Part model, mm, in its own coordinate system. Round coordinates to 2 decimals unless told otherwise and drop trailing zeros. Write each loop counter-clockwise with the first axis right and the second up, starting at its lowest first coordinate (ties: lowest second). Pieces come first, ordered by that corner, then holes. Notation, with made-up numbers: M 32,83 L 58,83 A27 ccw 58,119 Z; hole C -39,-8.5 d6. An arc over 180 degrees is marked long. One line per question, with ' | ' between items. Start each with the question number.
1) Saw through at B-B (y = 0). List the corners of the cut face in (x, z), plus the area to 3 significant figures.
2) Drop flat-ended pins along their axis: pin 1 Ø3 at (x, y) = (0.5, 2) entering from +Z; pin 2 Ø2 at (y, z) = (-1.5, -16.5) entering from +X; pin 3 Ø2 at (y, z) = (2, -14.5) entering from +X. Give the stop position or say it passes through.
3) Mould opens along Y. For faces 1 (the face through (-3, 0, -2)), 2 (the face through (-0.042, 0.481, -1.526)), 3 (the face through (0, -2, -15)) say: pulls with the +Y half, pulls with the -Y half, needs draft (parallel to the pull), parting line crosses it, or undercut.
4) Saw through at A-A (z = 0). List the corners of the cut face in (x, y).
5) Saw through at C-C (x = 2.5). List the corners of the cut face in (y, z).
6) Wall check: probe 1 along Y at (x, z) = (-0.95, 0); probe 2 along X at (y, z) = (0, -14); probe 3 along Y at (x, z) = (1.75, -0.5). Give the ranges that are in metal, low to high. Write a range as [from, to].
7) Saw through at D-D (x = 0). List the corners of the cut face in (y, z).
```python
from build123d import *

# Parameters (mm, degrees)
F_0012_CYLINDER_SKETCH_R     = 2
F_0012_CYLINDER_DEPTH        = 24
F_0014_CYLINDER_SKETCH_R     = 4
F_0014_CYLINDER_DEPTH        = 6
F_0014_CYLINDER_ROTATE_ANGLE = 90
F_0016_CYLINDER_SKETCH_R     = 1.6
F_0016_CYLINDER_DEPTH        = 8
F_0016_CYLINDER_ROTATE_ANGLE = 90


with BuildPart() as part:
    # 0012_cylinder_Sketch → 0012_cylinder (new body)
    with BuildSketch(Plane.XY):
        Circle(F_0012_CYLINDER_SKETCH_R)
    extrude(amount=F_0012_CYLINDER_DEPTH)


with BuildPart() as part_1:
    # 0012_cylinder_Translate: moved
    add(part.part.moved(Location((0, 0, -27))))


with BuildPart() as body_2:
    # 0014_cylinder_Sketch → 0014_cylinder (new body)
    with BuildSketch(Plane.XY):
        Circle(F_0014_CYLINDER_SKETCH_R)
    extrude(amount=F_0014_CYLINDER_DEPTH)


with BuildPart() as body_2_1:
    # 0014_cylinder_Rotate: moved
    add(body_2.part.rotate(Axis((0, 0, 0), (0, 1, 0)), F_0014_CYLINDER_ROTATE_ANGLE))


with BuildPart() as body_2_2:
    # 0014_cylinder_Translate: moved
    add(body_2_1.part.moved(Location((-3, 0, 0))))


with BuildPart() as part_2:
    add(part_1.part)

    # 0015_add: union body 2
    add(body_2_2.part)


with BuildPart() as body_2_2_1:
    # 0016_cylinder_Sketch → 0016_cylinder (new body)
    with BuildSketch(Plane.XY):
        Circle(F_0016_CYLINDER_SKETCH_R)
    extrude(amount=F_0016_CYLINDER_DEPTH)


with BuildPart() as body_2_2_2:
    # 0016_cylinder_Rotate: moved
    add(body_2_2_1.part.rotate(Axis((0, 0, 0), (0, 1, 0)), F_0016_CYLINDER_ROTATE_ANGLE))


with BuildPart() as body_2_2_3:
    # 0016_cylinder_Translate: moved
    add(body_2_2_2.part.moved(Location((-4, 0, 0))))


with BuildPart() as part_3:
    add(part_2.part)

    # 0017_sub: cut body 2 2
    add(body_2_2_3.part, mode=Mode.SUBTRACT)


solid = part_3.part
```
Answer key:
1) outline: M -3,-4 L -2,-4 L -2,-27 L 2,-27 L 2,-4 L 3,-4 L 3,-1.6 L -3,-1.6 Z; M -3,1.6 L 3,1.6 L 3,4 L -3,4 Z | area: 121 mm2
2) pin 1: stops at z = 3.97 | pin 2: stops at x = 1.94 | pin 3: stops at x = 1.73
3) face 1: needs draft | face 2: undercut | face 3: parting line crosses it
4) outline: M -3,-4 L 3,-4 L 3,-1.6 L -3,-1.6 Z; M -3,1.6 L 3,1.6 L 3,4 L -3,4 Z
5) outline: C 0,0 d8; hole C 0,0 d3.2
6) probe 1: y = [-4, -1.6], [1.6, 4] | probe 2: x = [-2, 2] | probe 3: y = [-3.97, -1.52], [1.52, 3.97]
7) outline: M -2,-27 L 2,-27 L 2,-3.46 A4 ccw long -2,-3.46 Z; hole C 0,0 d3.2
